Solid Edge part; units mm, degrees
sketch "Sketch1" plane through (0, 0, 0) normal (0, -1, 0) x (1, 0, 0)
  line L0 (28.9723, -16.0049) -> (28.9723, -4)
  line L1 (30.8556, 0.4736) -> (28.9723, -4)
  line L2 (41.8072, 11.4251) -> (30.8556, 0.4736)
  line L3 (53.9723, 11.4251) -> (41.8072, 11.4251)
  line L4 (53.9723, -16.0049) -> (53.9723, 11.4251)
  line L5 (28.9723, -16.0049) -> (53.9723, -16.0049)
extrude "Protrusion1" add sketch "Sketch1" against normal blind 95
sketch "Sketch2" plane through (53.9723, 47.5, 1.7845) normal (1, 0, 0) x (0, 1, 0)
  line L0 (39.1944, -10.7289) -> (40.75, -9.1733)
  line L1 (40.75, -9.1733) -> (42.3056, -10.7289)
  arc A0 (42.3056, -10.7289) -> (39.1944, -10.7289) centre (40.75, -12.2845) cw
  line L2 (-42.3056, -10.7289) -> (-40.75, -9.1733)
  line L3 (-40.75, -9.1733) -> (-39.1944, -10.7289)
  arc A1 (-39.1944, -10.7289) -> (-42.3056, -10.7289) centre (-40.75, -12.2845) cw
  dimension "D1" = 40.75
extrude "ExtrudedCutout_1" cut sketch "Sketch2" against normal blind 51.2416
sketch "Sketch3" plane through (41.4723, 0, -2.7874) normal (0, -1, 0) x (1, 0, 0)
  line L0 (2.8601, -0.8674) -> (2.8601, 15.2148)
  line L1 (2.8601, 15.2148) -> (-13.7847, 15.2148)
  line L2 (-13.7847, 15.2148) -> (-13.7847, -0.8674)
  line L3 (-13.7847, -0.8674) -> (2.8601, -0.8674)
extrude "ExtrudedCutout_12" cut sketch "Sketch3" against normal blind 115.4646
sketch "Sketch4" plane through (41.4723, 47.5, -17) normal (0, 0, -1) x (-1, 0, 0)
  line L0 (-6.1244, 32.9556) -> (-4.5754, 31.4066)
  line L1 (-4.5754, 31.4066) -> (-5.9875, 29.9945)
  arc A0 (-6.1244, 32.9556) -> (-5.9875, 29.9945) centre (-7.68, 31.4) ccw
  line L2 (-6.1244, 1.5556) -> (-4.5754, 0.0066)
  line L3 (-4.5754, 0.0066) -> (-6.2745, -1.6925)
  arc A1 (-6.1244, 1.5556) -> (-6.2745, -1.6925) centre (-7.68, 0) ccw
  line L4 (-6.0308, -29.944) -> (-4.5687, -31.6)
  line L5 (-4.5687, -31.6) -> (-6.2308, -33.0552)
  arc A2 (-6.0308, -29.944) -> (-6.2308, -33.0552) centre (-7.68, -31.4) ccw
extrude "ExtrudedCutout_14" cut sketch "Sketch4" against normal blind 69.6341
sketch "Sketch5" plane through (28.9723, 47.5, -10.5) normal (-1, 0, 0) x (0, -1, 0)
  line L0 (-34.5, -6.5) -> (-34.5, 6.8451)
  line L1 (-34.5, 6.8451) -> (34.5, 6.8451)
  line L2 (34.5, 6.8451) -> (34.5, -6.5)
  line L3 (34.5, -6.5) -> (-34.5, -6.5)
extrude "Cutout1" cut sketch "Sketch5" against normal up to surface (15.3601 mm away)
sketch "Sketch6" plane through (53.9723, 47.5, -2.7874) normal (1, 0, 0) x (0, 1, 0)
  line L0 (-17.5, -2.7126) -> (-17.5, 14.2126)
  line L1 (-17.5, 14.2126) -> (-47.5, 14.2126)
  line L2 (-47.5, 14.2126) -> (-47.5, -2.7126)
  line L3 (-47.5, -2.7126) -> (-37.5, -2.7126)
  line L4 (-37.5, -2.7126) -> (-17.5, -2.7126)
  line L5 (17.5, 14.2126) -> (17.5, -2.7126)
  line L6 (17.5, -2.7126) -> (37.5, -2.7126)
  line L7 (37.5, -2.7126) -> (47.5, -2.7126)
  line L8 (47.5, 14.2126) -> (47.5, -2.7126)
  line L9 (47.5, 14.2126) -> (17.5, 14.2126)
extrude "ExtrudedCutout_18" cut sketch "Sketch6" against normal blind 89.0785
sketch "Sketch7" plane through (53.9723, 47.5, -2.2899) normal (1, 0, 0) x (0, 1, 0)
  circle A0 centre (21.0894, -3.2101) radius 4.5049
  circle A1 centre (-21.933, -3.2101) radius 4.5049
  dimension "D1" = 21.933
extrude "Cutout2" cut sketch "Sketch7" against normal up to vertex (21.3514 mm away)
properties material "ABS Plastic, high impact"
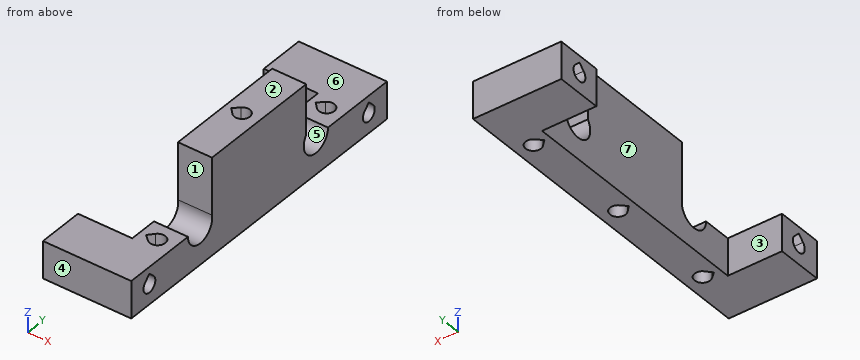
CAD build for the part. Positions are in the model's coordinates, mm. Face numbers are marked on the shaded views. A direction names the side the tool comes from. Round coordinates to 2 decimals unless told otherwise and drop trailing zeros. Order: outer loops, then holes, each group sorted by start corner. A loop starts at its lowest first (then second) coordinate and runs counter-clockwise, first axis right, second up. Notation, with made-up numbers: (69.5, 73.5) -> (90.5, 73.5) arc R7 cw to (90.5, 86.5) -> close; hole circle Ø10 at (-18.5, -10). An arc over 180 degrees is marked (long way). Write item = value, one per line. Start each with the question number.
(1) Pin check, flat tips, straight feed: P1, Ø5, axis at y = 68, z = -11, coming from the -X side; P2, Ø3, axis at x = 49, z = 2, coming from the -Y side; P3, Ø5, axis at x = 48, z = 6.5, coming from the +Y side. Stop position of each tip, or through.
(2) Which spindle directions (+Z, -Z, +X, -X, +Y, -Y) get a long thin tool onto all of the face, cutting with end or side? Do the marked faces 1, 2 and 3. Say none if no direction does.
(3) Cut at A-A, the plane x = 36.75. List the corners of the cut face in (y, z).
(4) Cut at C-C, the plane z = 8.5. List the corners of the cut face in (x, y), then the cut area to 3 significant figures.
(5) Pull direction Y, two halves, no side cores. Call the marked faces 4, 5, 6 and 7: released by +Y, released by -Y, zero draft, split by the parting line, or undercut.
(6) Probe line 1 (Y direction, x = 37, z = -10.5); line 2 (Y direction, x = 33.75, z = -14); line 3 (Y direction, x = 40, z = -8.25). List the from-to ranges inside material, lowest first. Write a range as [from, to].
(7) Cut at B-B, the plane z = -13.75. List the corners of the cut face in (x, y).
(8) Cut at D-D, the plane y = 35.5. List the corners of the cut face in (x, z), then the cut area to 3 significant figures.
Model answer:
q1.P1 = 44.33
q1.P2 = 30
q1.P3 = 65
q2.face_1 = +Z, +X, -X, -Y
q2.face_2 = +Z, +X, -X, +Y, -Y
q2.face_3 = +Z, -Z, -X
q3.outline = (0, -16) -> (13, -16) -> (13, -5.5) -> (0, -5.5) -> close; (82, -16) -> (95, -16) -> (95, -5.5) -> (82, -5.5) -> close; hole (5.19, -8.94) arc R2.2 ccw (long way) to (8.31, -8.94) -> (6.75, -7.39) -> close; hole (86.69, -8.94) arc R2.2 ccw (long way) to (89.81, -8.94) -> (88.25, -7.39) -> close
q4.outline = (44.33, 30) -> (53.97, 30) -> (53.97, 65) -> (44.33, 65) -> close; hole (46.05, 47.51) -> (47.75, 45.81) arc R2.2 ccw (long way) to (47.6, 49.06) -> close
q4.area = 321 mm2
q5.face_4 = released by -Y
q5.face_5 = undercut
q5.face_6 = zero draft
q5.face_7 = undercut
q6.line_1 = [0, 4.55], [8.95, 13], [82, 86.05], [90.45, 95]
q6.line_2 = [0, 13], [82, 95]
q6.line_3 = [0, 5.89], [7.61, 13], [82, 87.39], [89.11, 95]
q7.outline = (28.97, 0) -> (53.97, 0) -> (53.97, 95) -> (28.97, 95) -> (28.97, 82) -> (44.33, 82) -> (44.33, 13) -> (28.97, 13) -> close; hole (46.04, 15.9) -> (47.7, 14.44) arc R2.2 ccw (long way) to (47.5, 17.56) -> close; hole (46.05, 47.51) -> (47.75, 45.81) arc R2.2 ccw (long way) to (47.6, 49.06) -> close; hole (46.05, 78.91) -> (47.46, 77.49) arc R2.2 ccw (long way) to (47.6, 80.46) -> close
q8.outline = (44.33, -16) -> (53.97, -16) -> (53.97, 11.43) -> (44.33, 11.43) -> close
q8.area = 264 mm2
